Design review of the part built by this model. Coordinates are the model's own, in mm. A direction names the side the tool comes from. Give positions to 0.01 mm unless a question says otherwise; leave off trailing zeros. Loops run counter-clockwise (first coordinate to the right, second up) from the corner with the lowest first, then second, coordinate; pieces in that order, holes last. Notation, with made-up numbers: M 39.25,43.25 L 73.25,43.25 A29 ccw 73.25,81.25 Z; hole C 39,-31.5 d2. An arc over 180 degrees is marked long. Use CSV: the item, a comma, the result in double quotes.
from build123d import *

# Parameters (mm, degrees)
F0_W       = 5
F0_H       = 16
F0_W_2     = 12
F0_H_2     = 30
F0_H_3     = 20
F1_DEPTH   = 5
F0_H_4     = 102
F2_DEPTH   = 135
F3_SIZE2   = 35
F3_SIZE    = 100
F3_2_SIZE2 = 35
F3_2_SIZE  = 100
F5_D       = 20.5


with BuildPart() as f1:
    # F0 (on Top) → F1 (new body)
    with BuildSketch(Plane.XY):
        Polygon((29, 35), (29, 51), (-46, 51), (-46, -51), (29, -51), (29, -35), (29, -15), (29, 15), align=None)
        with Locations((31.5, 43)):
            Rectangle(F0_W, F0_H)
        with Locations((40, 43)):
            Rectangle(F0_W_2, F0_H)
        with Locations((31.5, 0)):
            Rectangle(F0_W, F0_H_2)
        with Locations((40, 0)):
            Rectangle(F0_W_2, F0_H_2)
        with Locations((31.5, -43)):
            Rectangle(F0_W, F0_H)
        with Locations((40, -25)):
            Rectangle(F0_W_2, F0_H_3)
        with Locations((40, 25)):
            Rectangle(F0_W_2, F0_H_3)
        Polygon((51, -51), (51, -35), (46, -35), (34, -35), (34, -51), align=None)
        with Locations((48.5, 43)):
            Rectangle(F0_W, F0_H)
        with Locations((48.5, 0)):
            Rectangle(F0_W, F0_H_2)
    extrude(amount=F1_DEPTH)

    # F0 (on Top) → F2 (join)
    with BuildSketch(Plane.XY):
        with Locations((-48.5, 0)):
            Rectangle(F0_W, F0_H_4)
    extrude(amount=F2_DEPTH)

    # F3
    f3_edges = [f1.edges().sort_by_distance(p)[0] for p in [
        (-48.5, -51, 135),
    ]]
    f3_side = f1.faces().sort_by_distance((49.307989, -51, 2.5))[0]
    chamfer(f3_edges, length=F3_SIZE, length2=F3_SIZE2, reference=f3_side)

    # F3#2
    f3_2_edges = [f1.edges().sort_by_distance(p)[0] for p in [
        (-48.5, 51, 135),
    ]]
    f3_2_side = f1.faces().sort_by_distance((49.307989, 51, 2.5))[0]
    chamfer(f3_2_edges, length=F3_2_SIZE, length2=F3_2_SIZE2, reference=f3_2_side)

    # F5 (through all)
    with Locations(Plane(origin=(-51, 0, 0), x_dir=(0, -1, 0), z_dir=(-1, 0, 0))):
        with Locations((0, 80)):
            Hole(F5_D / 2)


solid = f1.part
(1) We need section C-C on y = 32.5. State the section outline as (x, z) points.
A:
outline,"M -51,0 L 29,0 L 29,5 L -46,5 L -46,87.86 L -51,87.86 Z; M 34,0 L 46,0 L 46,5 L 34,5 Z"
(2) Clearance check with flat-ended pins moving along their axes: P1, Ø2.5, axis at y = 26.5, z = 2.5, coming from the +X side; P2, Ø5, axis at y = 17, z = 35.5, coming from the +X side; P3, Ø1.5, axis at x = -1.5, y = 22.5, coming from the +Z side. State where each tip first meets the part, or that it passes through.
A:
P1,"x = 46"
P2,"x = -46"
P3,"z = 5"
(3) We need section B-B on y = 0. State the section outline as (x, z) points, then the cut area to 3 significant figures.
A:
outline,"M -51,0 L 51,0 L 51,5 L -46,5 L -46,69.75 L -51,69.75 Z; M -51,90.25 L -46,90.25 L -46,135 L -51,135 Z"
area,"1,060 mm²"
(4) The part is to be moulded in two halves that separate along Y. For faces 4 (the flat face through (-8, 51, 4)), 5 (the flat face through (-48.535, -33.255, 85.7)), 6 (the flat face through (2, 1, 5)), 7 (the flat face through (34, 25, 2)), say which applies: released by +Y, released by -Y, zero draft, split by the parting line, or undercut.
A:
face 4,"released by +Y"
face 5,"released by -Y"
face 6,"zero draft"
face 7,"undercut"
(5) Machinability: for faces 1 (the flat face through (31, -35, 2)), 2 (the flat face through (-8, -51, 4)), 3 (the flat face through (46, 25, 2)), which of the approach directions +Z, -Z, +X, -X, +Y, -Y give a long, thin tool a straight path to every point of the face, cutting with its end or side? Answer none if there is none.
A:
face 1,"+Z, -Z"
face 2,"+Z, -Z, +X, -X, -Y"
face 3,"+Z, -Z, +X"
(6) Wall thickness on line 1 along Z through (x, y) = (-49.8, 0); line 2 along X through (y, z) = (-23, 50); line 3 along Z through (x, y) = (-3, 6): over which ranges is each line inside the solid? List them lowest first. Write a range as [from, to].
A:
line 1,"[0, 69.75], [90.25, 135]"
line 2,"[-51, -46]"
line 3,"[0, 5]"
(7) We need section D-D on x = -8. State the section outline as (y, z) points.
A:
outline,"M -51,0 L 51,0 L 51,5 L -51,5 Z"
(8) We need section A-A on z = 80. State the section outline as (x, y) points, then the cut area to 3 significant figures.
A:
outline,"M -51,-35.25 L -46,-35.25 L -46,-10.25 L -51,-10.25 Z; M -51,10.25 L -46,10.25 L -46,35.25 L -51,35.25 Z"
area,"250 mm²"
